Input: part model. Units: mm. Frame: model coordinates. Face numbers are marked on the shaded views. A direction names the side the tool comes from. Coordinates: 2 decimals unless noted, no trailing zeros. Write each loop counter-clockwise with the first axis right and the second up, starting at its lowest first coordinate (ties: lowest second). Pieces come first, ordered by that corner, then holes. Notation, with made-up numbers: M 5,-24.75 L 49,-24.75 A29 ccw 49,3.25 Z; hole C 51,17.25 d5. An arc over 180 degrees is marked long. Use one line per item in the form item = value.
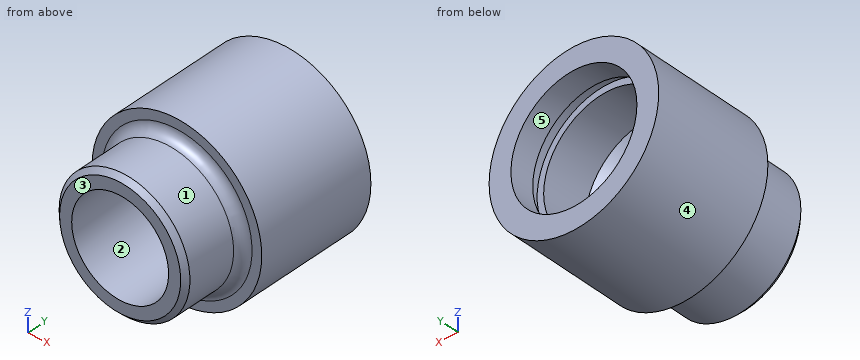
Autodesk Inventor part; units mm, degrees
ref_plane "YZ Plane" through (0, 0, 0) normal (1, 0, 0) x (0, 1, 0)
ref_plane "XZ Plane" through (0, 0, 0) normal (0, 1, 0) x (-1, 0, 0)
ref_plane "XY Plane" through (0, 0, 0) normal (0, 0, 1) x (1, 0, 0)
sketch "Sketch1" plane through (0, 0, 0) normal (0, 0, 1) x (1, 0, 0)
  line L0 (0, 0) -> (-13.5, 0)
  line L1 (-13.5, 0) -> (-13.5, 13)
  line L2 (-13.5, 13) -> (-17.5, 13)
  line L3 (-17.5, 13) -> (-17.5, 38)
  line L4 (-17.5, 38) -> (-13, 38)
  line L5 (-13, 38) -> (-13, 33)
  line L6 (-13, 33) -> (-14.35, 33)
  line L7 (-14.35, 33) -> (-14.35, 30.5)
  line L8 (-14.35, 30.5) -> (-13, 30.5)
  line L9 (-13, 30.5) -> (-13, 18)
  line L10 (-13, 18) -> (-10, 18)
  line L11 (-10, 18) -> (-10, 0)
  line L12 (0, 0) -> (0, 38)
  dimension "d0" = 13.5
  dimension "d1" = 13
  dimension "d2" = 4
  dimension "d3" = 25
  dimension "d4" = 4.5
  dimension "d5" = 5
  dimension "d6" = 1.35
  dimension "d7" = 2.5
  dimension "d8" = 12.5
  dimension "d9" = 3
revolve "Revolution1" add sketch "Sketch1" angle 360 about axis through (0, 0, 0) along (0, 1, 0)
fillet "Fillet1" radius 2 1 edges at (13.5, 13, 0)
chamfer "Chamfer1" distance 3 angle 45 1 edges at (13, 18, 0)
chamfer "Chamfer2" distance 1 angle 45 1 edges at (13.5, 0, 0)
thread "Thread1"
properties part number "Heated tube-transfer tube connector" material "Polypropylene"
(1) Pull-direction query (Z, two-part tool) for the marked faces 1, 2 and 3; classes: pulls with the +Z half, pulls with the -Z half, needs draft (parallel to the pull), parting line crosses it, or undercut.
Computed:
face_1 = parting line crosses it
face_2 = undercut
face_3 = needs draft
(2) Section query C-C on y = 10. Return the cut outline in (x, z), plus the area to 3 significant figures.
Computed:
outline = C 0,0 d27; hole C 0,0 d20
area = 258 mm^2
(3) First-contact query: pin 1 Ø4 at (x, z) = (7.5, 5.5) entering from -Y; pin 2 Ø8 at (x, z) = (6, -5) entering from +Y; pin 3 Ø5 at (y, z) = (30.5, 12) entering from +X; pin 4 Ø8 at (x, y) = (8, 28) entering from +Z. Flat tips, straight axial feed; report the tip coordinate or a pass-through.
Computed:
pin_1 = 0
pin_2 = 19.81
pin_3 = 14.7
pin_4 = 17.04
(4) Set-up query: the marked faces 4 and 5. Return all of +Z, -Z, +X, -X, +Y, -Y with unobstructed straight access to the full face (end or side cutting, diameter ignored); none if empty.
Computed:
face_4 = +Y, -Y
face_5 = +Y
(5) Line query: probe 1 along Z at (x, y) = (0, 35.8); probe 2 along Z at (x, y) = (-7, 36); probe 3 along Y at (x, z) = (13, -5.5). Output: solid intervals per line, ascending.
Computed:
probe_1 = -17.5 to -13, 13 to 17.5
probe_2 = -16.04 to -10.95, 10.95 to 16.04
probe_3 = 12.44 to 30.5, 33 to 38
(6) Section query D-D on y = 17. Return the cut outline in (x, z).
Computed:
outline = C 0,0 d35; hole C 0,0 d20
